Geometry check sheet. Reference: the model listing, model coordinates, mm. Face numbers are marked on the shaded views. A direction names the side the tool comes from. Round coordinates to 2 decimals unless told otherwise and drop trailing zeros. Order: outer loops, then holes, each group sorted by start corner. A loop starts at its lowest first (then second) coordinate and runs counter-clockwise, first axis right, second up.
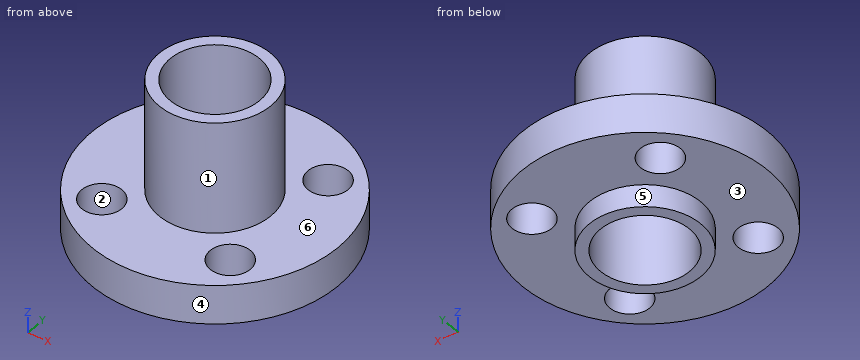
```python
from build123d import *

# Parameters (mm, degrees)
SKETCH_R     = 11
SKETCH_R_2   = 1.8
PAD_DEPTH    = 3.5
SKETCH001_R  = 5
PAD001_DEPTH = 10
SKETCH002_R  = 5
PAD002_DEPTH = 2
SKETCH003_R  = 4
POCKET_DEPTH = 15.5


with BuildPart() as part:
    # Sketch → Pad (new body)
    with BuildSketch(Plane.XY):
        Circle(SKETCH_R)
        with Locations((-5.75, 5.75)):
            Circle(SKETCH_R_2, mode=Mode.SUBTRACT)
        with Locations((5.75, 5.75)):
            Circle(SKETCH_R_2, mode=Mode.SUBTRACT)
        with Locations((5.75, -5.75)):
            Circle(SKETCH_R_2, mode=Mode.SUBTRACT)
        with Locations((-5.75, -5.75)):
            Circle(SKETCH_R_2, mode=Mode.SUBTRACT)
    extrude(amount=PAD_DEPTH)

    # Sketch001 → Pad001 (new body)
    with BuildSketch(Plane.XY.offset(3.5)):
        Circle(SKETCH001_R)
    extrude(amount=PAD001_DEPTH)

    # Sketch002 → Pad002 (new body)
    with BuildSketch(Plane(origin=(0, 0, 0), x_dir=(1, 0, 0), z_dir=(0, 0, -1))):
        Circle(SKETCH002_R)
    extrude(amount=PAD002_DEPTH)

    # Sketch003 → Pocket (cut)
    with BuildSketch(Plane(origin=(0, 0, -2), x_dir=(1, 0, 0), z_dir=(0, 0, -1))):
        Circle(SKETCH003_R)
    extrude(amount=-POCKET_DEPTH, mode=Mode.SUBTRACT)


solid = part.part
```
(1) Sectioned sample at D-D, the plane y = 5.75. Record the cut outline in (x, z).
Returned:
outline: (-9.38, 0) - (-7.55, 0) - (-7.55, 3.5) - (-9.38, 3.5) - close; (-3.95, 0) - (3.95, 0) - (3.95, 3.5) - (-3.95, 3.5) - close; (7.55, 0) - (9.38, 0) - (9.38, 3.5) - (7.55, 3.5) - close
(2) Sectioned sample at B-B, the plane z = 0.5. Record the cut outline in (x, y).
Returned:
outline: circle Ø22 at (0, 0); hole circle Ø3.6 at (-5.75, -5.75); hole circle Ø3.6 at (-5.75, 5.75); hole circle Ø8 at (0, 0); hole circle Ø3.6 at (5.75, -5.75); hole circle Ø3.6 at (5.75, 5.75)
(3) Material ranges on line 1 (Y direction, x = 0, z = 9); line 2 (Y direction, x = -5.75, z = 2.65); line 3 (Z direction, x = 6.5, y = -0.75), recorded low to high.
Returned:
line 1: y = -5 to -4, 4 to 5
line 2: y = -9.38 to -7.55, -3.95 to 3.95, 7.55 to 9.38
line 3: z = 0 to 3.5
(4) Depth check by flat-ended pin: P1, Ø6, axis at x = 1.5, y = 7, coming from the +Z side; P2, Ø4.5, axis at x = -5.75, y = -5.75, coming from the -Z side; P3, Ø1, axis at y = 4, z = 9.5, coming from the +X side; P4, Ø4.5, axis at x = -5.75, y = 5.75, coming from the +Z side. Enter the tip coordinate at first touch or a pass-through.
Returned:
P1: stops at z = 13.5
P2: stops at z = 0
P3: stops at x = 3.57
P4: stops at z = 3.5
(5) Sectioned sample at A-A, the plane y = 0. Record the cut outline in (x, z), and give its area (3 significant figures).
Returned:
outline: (-11, 0) - (-5, 0) - (-5, -2) - (-4, -2) - (-4, 13.5) - (-5, 13.5) - (-5, 3.5) - (-11, 3.5) - close; (4, -2) - (5, -2) - (5, 0) - (11, 0) - (11, 3.5) - (5, 3.5) - (5, 13.5) - (4, 13.5) - close
area: 73.0 mm2
(6) Draft check along Y on the marked faces 1, 2 and 3. Enter one of: released by +Y, released by -Y, zero draft, split by the parting line, or undercut.
Returned:
face 1: split by the parting line
face 2: undercut
face 3: zero draft
(7) Set-up check for the marked faces 4, 5 and 6: record each of +Z, -Z, +X, -X, +Y, -Y from which the full face is reachable in a straight line by a thin tool's end or side.
Returned:
face 4: +Z, -Z
face 5: -Z
face 6: +Z
